Design review of the part built by this model. Coordinates are the model's own, in mm. A direction names the side the tool comes from. Round coordinates to 2 decimals unless told otherwise and drop trailing zeros. Loops run counter-clockwise (first coordinate to the right, second up) from the corner with the lowest first, then second, coordinate; pieces in that order, holes last. Notation, with made-up numbers: (19, 72) -> (78, 72) arc R31 ccw to (78, 99) -> close; hole circle Ø7 at (3, 36.25). An arc over 180 degrees is marked (long way). Answer as CSV lines item,"result". Start each with the question number.
(1) Take a section at C-C, the plane x = -88.9. Write out the cut boundary in (y, z) (3 decimals).
(2) For P1, Ø4, axis at x = -88.9, z = 0, coming from the -Y side; P2, Ø5, axis at x = 68, z = 62.5, coming from the -Y side, all flat-tipped, find the tip position at first contact; note any pin that passes through.
(3) Take a section at D-D, the plane x = 88.5. Write out the cut boundary in (y, z) (3 decimals), and give its area (3 significant figures).
(4) Machinability: for faces 1 (the face through (-92.07, 1.61, -0.14)), 2 (the face through (-1, 3.175, -1)), which of the approach directions +Z, -Z, +X, -X, +Y, -Y give a long, thin tool a straight path to every point of the face, cutting with its end or side? Answer none if there is none.
(5) To check wall thickness, follow line 1 (X direction, y = 3.5, z = -2); line 2 (X direction, y = 1, z = 0) (3 decimals); line 3 (Z direction, x = -88.9, y = 1.6) (3 decimals). State the ranges of each line that lie inside material, in increasing order. Write a range as from..to.
(6) Draft analysis for pull direction Z (two halves, no side actions). For faces 3 (the face through (-127, 3, 1)), 4 (the face through (-24.71, 4.74, 39.76)), 5 (the face through (-22.478, 4.74, -40.133)), 6 (the face through (-2, 3, 101.6)), state which applies: +Z half, -Z half, draft (parallel to the pull), parting line (faces both ways), or undercut.
(7) Take a section at B-B, the plane y = 5. Write out the cut boundary in (x, z) (3 decimals).
(8) Take a section at A-A, the plane z = 0. Write out the cut boundary in (x, y) (3 decimals), and give its area (3 significant figures).
from build123d import *

# Parameters (mm, degrees)
SKETCH1_W           = 254
SKETCH1_H           = 203.2
BOSS_EXTRUDE1_DEPTH = 6.35
SKETCH2_R           = 3.175
CUT_EXTRUDE1_DEPTH  = 6.35
CUT_EXTRUDE3_DEPTH  = 3.175
FILLET2_R           = 304.8


with BuildPart() as part:
    # Sketch1 → Boss-Extrude1 (new body)
    with BuildSketch(Plane(origin=(0, 0, 0), x_dir=(1, 0, 0), z_dir=(0, 1, 0))):
        Rectangle(SKETCH1_W, SKETCH1_H)
    extrude(amount=BOSS_EXTRUDE1_DEPTH)

    # Sketch2 → Cut-Extrude1 (cut)
    with BuildSketch(Plane(origin=(0, 6.35, 0), x_dir=(1, 0, 0), z_dir=(0, 1, 0))):
        with Locations((-88.9, 0)):
            Circle(SKETCH2_R)
    extrude(amount=-CUT_EXTRUDE1_DEPTH, mode=Mode.SUBTRACT)

    # Sketch5 → Cut-Extrude3 (cut)
    with BuildSketch(Plane(origin=(0, 6.35, 0), x_dir=(1, 0, 0), z_dir=(0, 1, 0))):
        Polygon((-101.6, 15.875), (-101.6, -15.875), (-25.4, -50.8), (101.6, -38.1), (101.6, 38.1), (-25.4, 50.8), align=None)
    extrude(amount=-CUT_EXTRUDE3_DEPTH, mode=Mode.SUBTRACT)

    # Fillet2
    fillet2_edges = [part.edges().sort_by_distance(p)[0] for p in [
        (-25.4, 4.7625, -50.8),
        (-25.4, 4.7625, 50.8),
    ]]
    fillet(fillet2_edges, radius=FILLET2_R)


solid = part.part
The answers:
1,outline,"(0, -101.6) -> (6.35, -101.6) -> (6.35, -21.407) -> (3.175, -21.407) -> (3.175, -3.175) -> (0, -3.175) -> close; (0, 3.175) -> (3.175, 3.175) -> (3.175, 21.407) -> (6.35, 21.407) -> (6.35, 101.6) -> (0, 101.6) -> close"
2,P1,"through"
2,P2,"y = 0"
3,outline,"(0, -101.6) -> (6.35, -101.6) -> (6.35, -39.41) -> (3.175, -39.41) -> (3.175, 39.41) -> (6.35, 39.41) -> (6.35, 101.6) -> (0, 101.6) -> close"
3,area,"1,040 mm²"
4,face 1,"+Y, -Y"
4,face 2,"+Y"
5,line 1,"-127..-101.6, 101.6..127"
5,line 2,"-127..-92.075, -85.725..127"
5,line 3,"-101.6..-3.175, 3.175..101.6"
6,face 3,"draft"
6,face 4,"undercut"
6,face 5,"undercut"
6,face 6,"+Z half"
7,outline,"(-127, -101.6) -> (127, -101.6) -> (127, 101.6) -> (-127, 101.6) -> close; hole (-101.6, -15.875) -> (-100.511, -16.374) arc R304.8 ccw to (56.814, -42.579) -> (101.6, -38.1) -> (101.6, 38.1) -> (56.814, 42.579) arc R304.8 ccw to (-100.511, 16.374) -> (-101.6, 15.875) -> close"
8,outline,"(-127, 0) -> (-92.075, 0) -> (-92.075, 3.175) -> (-101.6, 3.175) -> (-101.6, 6.35) -> (-127, 6.35) -> close; (-85.725, 0) -> (127, 0) -> (127, 6.35) -> (101.6, 6.35) -> (101.6, 3.175) -> (-85.725, 3.175) -> close"
8,area,"948 mm²"
